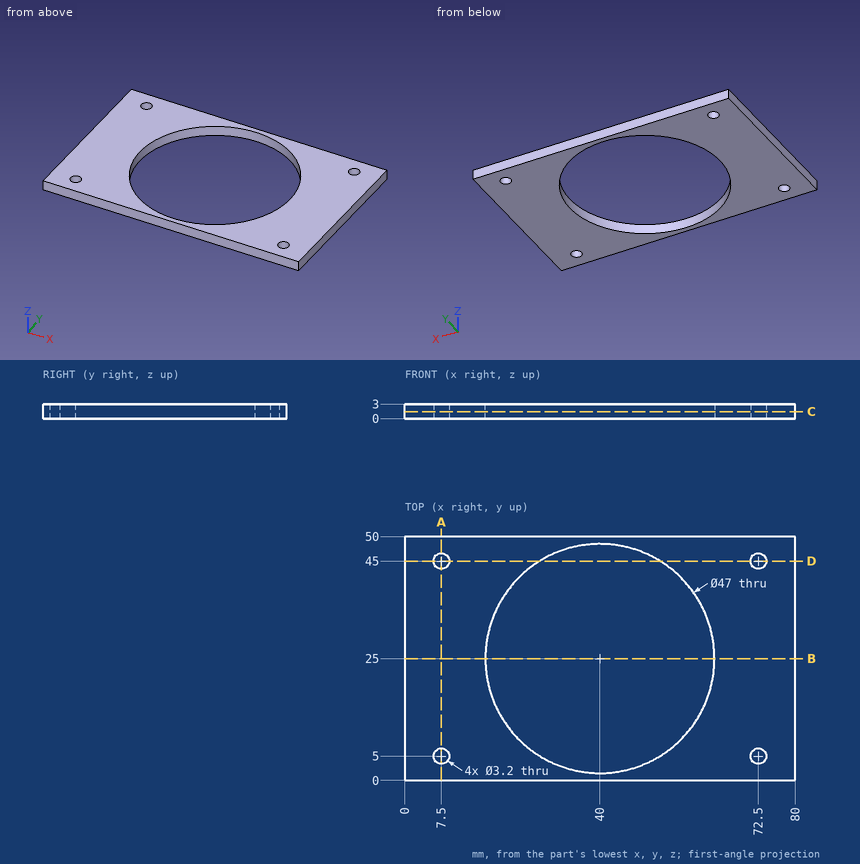
Verification items for this drawing (mm, ordinates from the low corner). Give positions to 0.01 mm unless a question says otherwise; leave off trailing zeros. Loops run counter-clockwise (first coordinate to the right, second up) from the corner with the lowest first, then second, coordinate; pieces in that order, holes last. Notation, with made-up numbers: M 14.25,67.5 L 37.25,67.5 A23 ccw 37.25,87.5 Z; hole C 1.5,-19 d8. An arc over 180 degrees is marked long. Answer as CSV lines item,"result".
Item 1: Cross-section at C-C on z = 1.45. Record the cut outline in (x, y).
Values:
outline,"M 0,0 L 80,0 L 80,50 L 0,50 Z; hole C 7.5,5 d3.2; hole C 7.5,45 d3.2; hole C 40,25 d47; hole C 72.5,5 d3.2; hole C 72.5,45 d3.2"
Item 2: Depth check by flat-ended pin: P1, Ø2, axis at x = 61, y = 22.5, coming from the +Z side. Enter the tip coordinate at first touch or a pass-through.
Values:
P1,"passes through"
Item 3: Cross-section at B-B on y = 25. Record the cut outline in (x, z), and give its area (3 significant figures).
Values:
outline,"M 0,0 L 16.5,0 L 16.5,3 L 0,3 Z; M 63.5,0 L 80,0 L 80,3 L 63.5,3 Z"
area,"99.0 mm²"
Item 4: Material ranges on line 1 (Y direction, x = 72.5, z = 1.05); line 2 (Y direction, x = 72, z = 1.45); line 3 (X direction, y = 5, z = 1.5), recorded low to high.
Values:
line 1,"y = 0 to 3.4, 6.6 to 43.4, 46.6 to 50"
line 2,"y = 0 to 3.48, 6.52 to 43.48, 46.52 to 50"
line 3,"x = 0 to 5.9, 9.1 to 27.66, 52.34 to 70.9, 74.1 to 80"
Item 5: Cross-section at D-D on y = 45. Record the cut outline in (x, z).
Values:
outline,"M 0,0 L 5.9,0 L 5.9,3 L 0,3 Z; M 9.1,0 L 27.66,0 L 27.66,3 L 9.1,3 Z; M 52.34,0 L 70.9,0 L 70.9,3 L 52.34,3 Z; M 74.1,0 L 80,0 L 80,3 L 74.1,3 Z"
Item 6: Cross-section at A-A on x = 7.5. Record the cut outline in (y, z).
Values:
outline,"M 0,0 L 3.4,0 L 3.4,3 L 0,3 Z; M 6.6,0 L 43.4,0 L 43.4,3 L 6.6,3 Z; M 46.6,0 L 50,0 L 50,3 L 46.6,3 Z"
